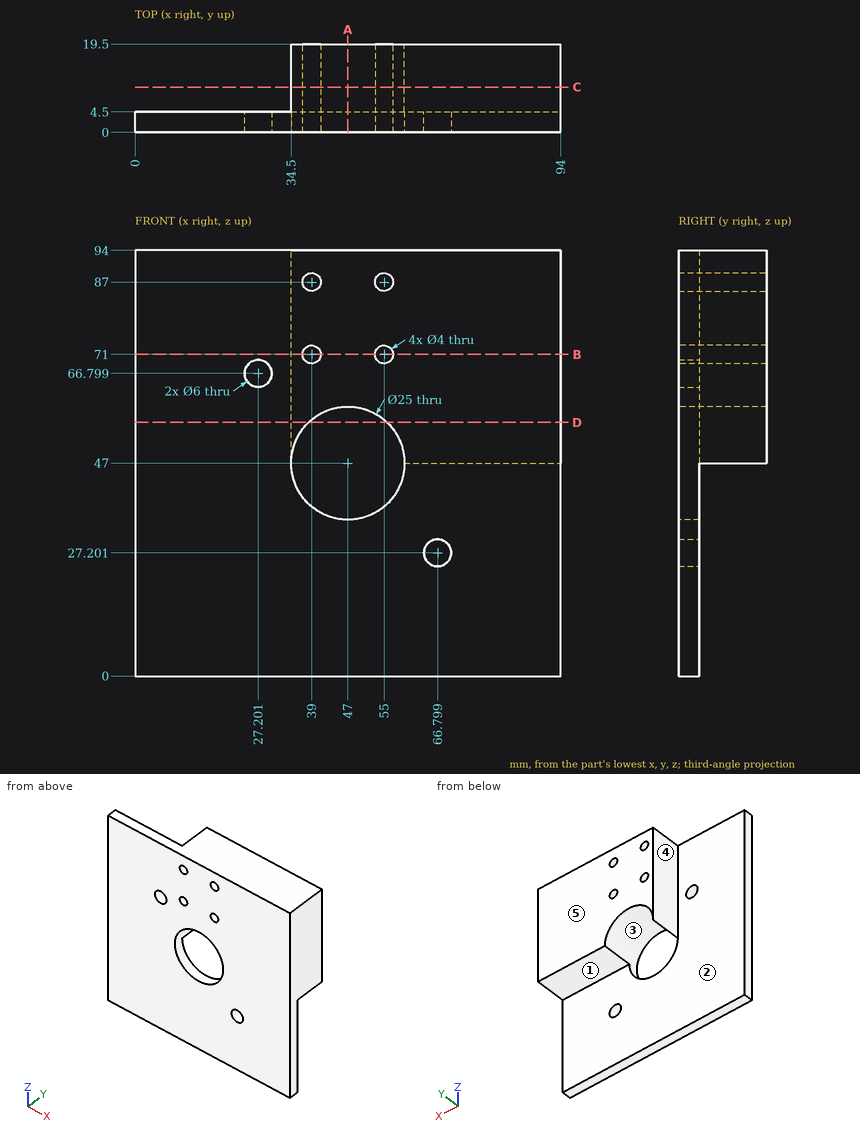
Input: dimensioned drawing with shaded views. Units: mm. Origin: part minimum x, y, z. A direction names the side the tool comes from. Coordinates: 2 decimals unless noted, no trailing zeros. Order: outer loops, then holes, each group sorted by start corner. A loop starts at its lowest first (then second) coordinate and runs counter-clockwise, first axis right, second up.
(1) Section query C-C (y = 10). Return the cut outline in (x, z).
(2) Access query for the marked faces 4 and 5. Directions: +Z, -Z, +X, -X, +Y, -Y. A direction counts if a zero-diameter tool reaches every point of the face in a straight line with its end or side. Return the directions, or none.
(3) Section query D-D (z = 56). Return the cut outline in (x, y).
(4) First-contact query: pin 1 (6 mm diameter, centred on x = 81, y = 12.5, fed in from -Z); pin 2 (4.5 mm diameter, centred on x = 39, z = 71, fed in from +Y); pin 3 (10 mm diameter, centred on x = 84, z = 20, fed in from +Y); pin 4 (7.5 mm diameter, centred on y = 15, z = 68, fed in from -X). Flat tips, straight axial feed; report the tip coordinate or a pass-through.
(5) Material intervals for probe 1 along X at (y, z) = (15.5, 87); probe 2 along Z at (x, y) = (40.5, 10.5); probe 3 along Y at (x, z) = (7, 69), sorted ascending.
(6) Section query B-B (z = 71). Return the cut outline in (x, y).
(7) Draft query along Z for the marked faces 1, 2 and 3. Return one class per face: pulls with the +Z half, pulls with the -Z half, needs draft (parallel to the pull), parting line crosses it, or undercut.
(8) Section query A-A (x = 47). Return the cut outline in (y, z), plus the area to 3 significant figures.
Solution:
1. outline: (34.5, 47) arc R12.5 cw to (59.5, 47) - (94, 47) - (94, 94) - (34.5, 94) - close; hole circle Ø4 at (39, 71); hole circle Ø4 at (39, 87); hole circle Ø4 at (55, 71); hole circle Ø4 at (55, 87)
2. face 4: +Z, -Z, -X, +Y
2. face 5: +Z, -Z, +X, -X, +Y
3. outline: (0, 0) - (38.33, 0) - (38.33, 19.5) - (34.5, 19.5) - (34.5, 4.5) - (0, 4.5) - close; (55.67, 0) - (94, 0) - (94, 19.5) - (55.67, 19.5) - close
4. pin 1: stops at z = 47
4. pin 2: stops at y = 19.5
4. pin 3: stops at y = 4.5
4. pin 4: stops at x = 34.5
5. probe 1: x = 34.5 to 37, 41 to 53, 57 to 94
5. probe 2: z = 57.68 to 69.68, 72.32 to 85.68, 88.32 to 94
5. probe 3: y = 0 to 4.5
6. outline: (0, 0) - (37, 0) - (37, 19.5) - (34.5, 19.5) - (34.5, 4.5) - (0, 4.5) - close; (41, 0) - (53, 0) - (53, 19.5) - (41, 19.5) - close; (57, 0) - (94, 0) - (94, 19.5) - (57, 19.5) - close
7. face 1: pulls with the -Z half
7. face 2: needs draft
7. face 3: undercut
8. outline: (0, 0) - (4.5, 0) - (4.5, 34.5) - (0, 34.5) - close; (0, 59.5) - (19.5, 59.5) - (19.5, 94) - (0, 94) - close
8. area: 828 mm2
